```python
from build123d import *

# Parameters (mm, degrees)
SKETCH1_R           = 37
BOSS_EXTRUDE1_DEPTH = 3
SKETCH1_3_R         = 30
SKETCH1_3_R_2       = 14
BOSS_EXTRUDE2_DEPTH = 29
CUT_EXTRUDE1_START  = -4
SKETCH2_R           = 25
SKETCH2_R_2         = 23.5
CUT_EXTRUDE1_DEPTH  = 4
SKETCH3_R           = 4
SKETCH3_R_2         = 2
CUT_EXTRUDE2_DEPTH  = 4


with BuildPart() as part:
    # Sketch1 → Boss-Extrude1 (new body)
    with BuildSketch(Plane(origin=(0, 0, 0), x_dir=(1, 0, 0), z_dir=(0, 1, 0))):
        with Locations(Location((0, 0, 0), (0, 0, 270))):
            Circle(SKETCH1_R)
    extrude(amount=BOSS_EXTRUDE1_DEPTH)

    # Sketch1<3> → Boss-Extrude2 (add)
    with BuildSketch(Plane(origin=(0, 0, 0), x_dir=(1, 0, 0), z_dir=(0, 1, 0))):
        with Locations(Location((0, 0, 0), (0, 0, 90))):
            Circle(SKETCH1_3_R)
        with Locations(Location((0, 0, 0), (0, 0, 90))):
            Circle(SKETCH1_3_R_2, mode=Mode.SUBTRACT)
    extrude(amount=BOSS_EXTRUDE2_DEPTH)

    # Sketch2 → Cut-Extrude1 (cut)
    # profile 1 of 10: a face of its own
    with BuildSketch(Plane(origin=(0, 29, 0), x_dir=(1, 0, 0), z_dir=(0, 1, 0)).offset(CUT_EXTRUDE1_START)):
        with Locations(Location((0, 0, 0), (0, 0, 270))):
            Circle(SKETCH2_R)
        Circle(SKETCH2_R_2, mode=Mode.SUBTRACT)
    # profile 2 of 10: a face of its own
    with BuildSketch(Plane(origin=(0, 29, 0), x_dir=(1, 0, 0), z_dir=(0, 1, 0)).offset(CUT_EXTRUDE1_START)):
        with BuildLine():
            ThreePointArc((24.954959427, 1.5), (0, 25), (-24.954959427, 1.5))
            Line((-24.954959427, 1.5), (-23.452078799, 1.5))
            ThreePointArc((-23.452078799, 1.5), (0, 23.5), (23.452078799, 1.5))
            Line((23.452078799, 1.5), (24.954959427, 1.5))
        make_face()
    # profile 3 of 10: a face of its own
    with BuildSketch(Plane(origin=(0, 29, 0), x_dir=(1, 0, 0), z_dir=(0, 1, 0)).offset(CUT_EXTRUDE1_START)):
        with BuildLine():
            ThreePointArc((-24.954959427, 1.5), (-25, 0), (-24.954959427, -1.5))
            Line((-24.954959427, -1.5), (-23.452078799, -1.5))
            ThreePointArc((-23.452078799, -1.5), (-23.5, 0), (-23.452078799, 1.5))
            Line((-23.452078799, 1.5), (-24.954959427, 1.5))
        make_face()
    # profile 4 of 10: a face of its own
    with BuildSketch(Plane(origin=(0, 29, 0), x_dir=(1, 0, 0), z_dir=(0, 1, 0)).offset(CUT_EXTRUDE1_START)):
        with BuildLine():
            Line((23.452078799, -1.5), (24.954959427, -1.5))
            ThreePointArc((24.954959427, -1.5), (24.98873732, -0.750338033), (25, 0))
            ThreePointArc((25, 0), (24.98873732, 0.750338033), (24.954959427, 1.5))
            Line((24.954959427, 1.5), (23.452078799, 1.5))
            ThreePointArc((23.452078799, 1.5), (23.488016644, 0.750382643), (23.5, 0))
            ThreePointArc((23.5, 0), (23.488016644, -0.750382643), (23.452078799, -1.5))
        make_face()
    # profile 5 of 10: a face of its own
    with BuildSketch(Plane(origin=(0, 29, 0), x_dir=(1, 0, 0), z_dir=(0, 1, 0)).offset(CUT_EXTRUDE1_START)):
        with BuildLine():
            ThreePointArc((-23.452078799, 1.5), (-23.5, 0), (-23.452078799, -1.5))
            Line((-23.452078799, -1.5), (-13.919410907, -1.5))
            ThreePointArc((-13.919410907, -1.5), (-14, 0), (-13.919410907, 1.5))
            Line((-13.919410907, 1.5), (-23.452078799, 1.5))
        make_face()
    # profile 6 of 10: a face of its own
    with BuildSketch(Plane(origin=(0, 29, 0), x_dir=(1, 0, 0), z_dir=(0, 1, 0)).offset(CUT_EXTRUDE1_START)):
        with BuildLine():
            Line((13.919410907, -1.5), (23.452078799, -1.5))
            ThreePointArc((23.452078799, -1.5), (23.488016644, -0.750382643), (23.5, 0))
            ThreePointArc((23.5, 0), (23.488016644, 0.750382643), (23.452078799, 1.5))
            Line((23.452078799, 1.5), (13.919410907, 1.5))
            ThreePointArc((13.919410907, 1.5), (13.979838209, 0.751081654), (14, 0))
            ThreePointArc((14, 0), (13.979838209, -0.751081654), (13.919410907, -1.5))
        make_face()
    # profile 7 of 10: a face of its own
    with BuildSketch(Plane(origin=(0, 29, 0), x_dir=(1, 0, 0), z_dir=(0, 1, 0)).offset(CUT_EXTRUDE1_START)):
        with BuildLine():
            ThreePointArc((-23.452078799, 1.5), (-23.5, 0), (-23.452078799, -1.5))
            Line((-23.452078799, -1.5), (-13.919410907, -1.5))
            ThreePointArc((-13.919410907, -1.5), (-14, 0), (-13.919410907, 1.5))
            Line((-13.919410907, 1.5), (-23.452078799, 1.5))
        make_face()
    # profile 8 of 10: a face of its own
    with BuildSketch(Plane(origin=(0, 29, 0), x_dir=(1, 0, 0), z_dir=(0, 1, 0)).offset(CUT_EXTRUDE1_START)):
        with BuildLine():
            Line((13.919410907, -1.5), (23.452078799, -1.5))
            ThreePointArc((23.452078799, -1.5), (23.488016644, -0.750382643), (23.5, 0))
            ThreePointArc((23.5, 0), (23.488016644, 0.750382643), (23.452078799, 1.5))
            Line((23.452078799, 1.5), (13.919410907, 1.5))
            ThreePointArc((13.919410907, 1.5), (13.979838209, 0.751081654), (14, 0))
            ThreePointArc((14, 0), (13.979838209, -0.751081654), (13.919410907, -1.5))
        make_face()
    # profile 9 of 10: a face of its own
    with BuildSketch(Plane(origin=(0, 29, 0), x_dir=(1, 0, 0), z_dir=(0, 1, 0)).offset(CUT_EXTRUDE1_START)):
        with BuildLine():
            ThreePointArc((-24.954959427, 1.5), (-25, 0), (-24.954959427, -1.5))
            Line((-24.954959427, -1.5), (-23.452078799, -1.5))
            ThreePointArc((-23.452078799, -1.5), (-23.5, 0), (-23.452078799, 1.5))
            Line((-23.452078799, 1.5), (-24.954959427, 1.5))
        make_face()
    # profile 10 of 10: a face of its own
    with BuildSketch(Plane(origin=(0, 29, 0), x_dir=(1, 0, 0), z_dir=(0, 1, 0)).offset(CUT_EXTRUDE1_START)):
        with BuildLine():
            Line((23.452078799, -1.5), (24.954959427, -1.5))
            ThreePointArc((24.954959427, -1.5), (24.98873732, -0.750338033), (25, 0))
            ThreePointArc((25, 0), (24.98873732, 0.750338033), (24.954959427, 1.5))
            Line((24.954959427, 1.5), (23.452078799, 1.5))
            ThreePointArc((23.452078799, 1.5), (23.488016644, 0.750382643), (23.5, 0))
            ThreePointArc((23.5, 0), (23.488016644, -0.750382643), (23.452078799, -1.5))
        make_face()
    extrude(amount=CUT_EXTRUDE1_DEPTH, mode=Mode.SUBTRACT)

    # Sketch3 → Cut-Extrude2 (cut)
    with BuildSketch(Plane.XZ):
        with Locations(Location((0, 0, 0), (0, 0, 270))):
            Circle(SKETCH3_R)
        with Locations(Location((-8, 0, 0), (0, 0, 270))):
            Circle(SKETCH3_R_2)
        with Locations(Location((0, 8, 0), (0, 0, 270))):
            Circle(SKETCH3_R_2)
        with Locations(Location((8, 0, 0), (0, 0, 270))):
            Circle(SKETCH3_R_2)
        with Locations(Location((0, -8, 0), (0, 0, 270))):
            Circle(SKETCH3_R_2)
    extrude(amount=-CUT_EXTRUDE2_DEPTH, mode=Mode.SUBTRACT)


solid = part.part
```
The model under review builds one solid part; all positions refer to its coordinate system, in mm. A direction names the side the tool comes from. Give positions to 0.01 mm unless a question says otherwise; leave off trailing zeros. Write each loop counter-clockwise with the first axis right and the second up, starting at its lowest first coordinate (ties: lowest second). Pieces come first, ordered by that corner, then holes. Notation, with made-up numbers: (54, 2.5) -> (86, 2.5) arc R12 ccw to (86, 20.5) -> close; hole circle Ø10 at (32, 61.25). An arc over 180 degrees is marked (long way). Put each result on its own line as item: value.
(1) We need section C-C, the plane y = 19.5. Give the boundary of the cut face in (x, z), and give its area (3 significant figures).
Results are:
outline: circle Ø60 at (0, 0); hole circle Ø28 at (0, 0)
area: 2,210 mm²
(2) We need section D-D, the plane x = -8. Give the boundary of the cut face in (y, z), and give its area (3 significant figures).
Results are:
outline: (0, -36.12) -> (3, -36.12) -> (3, -28.91) -> (29, -28.91) -> (29, -23.69) -> (25, -23.69) -> (25, -22.1) -> (29, -22.1) -> (29, -11.49) -> (3, -11.49) -> (3, -2) -> (0, -2) -> close; (0, 2) -> (3, 2) -> (3, 11.49) -> (29, 11.49) -> (29, 22.1) -> (25, 22.1) -> (25, 23.69) -> (29, 23.69) -> (29, 28.91) -> (3, 28.91) -> (3, 36.12) -> (0, 36.12) -> close
area: 1,100 mm²
(3) The part is to be moulded in two halves that separate along X. For faces 3 (the cylindrical face through (-0.496, 26.972, 23.495)), 4 (the flat face through (-25, 29, 7)), 5 (the cylindrical face through (-14.17, 1.48, 34.18)), say which applies: pulls with the +X half, pulls with the -X half, needs draft (parallel to the pull), parting line crosses it, or undercut.
Results are:
face 3: undercut
face 4: needs draft
face 5: parting line crosses it
(4) For pin 1 Ø5 at (y, z) = (13.5, -16.5) entering from -X; pin 2 Ø8.5 at (x, z) = (-0.5, 3.5) entering from +Y; pin 3 Ø1 at (x, y) = (19, 20) entering from +Z, all flat-tipped, find the tip position at first contact; note any pin that passes through.
Results are:
pin 1: x = -26.53
pin 2: y = 3
pin 3: z = 23.62
(5) To check wall thickness, follow probe 1 along X at (y, z) = (0.7, 0); probe 2 along X at (y, z) = (15.5, 0); probe 3 along Z at (x, y) = (-4, 25.75). State the ranges of each line that lie inside material, in increasing order. Write a range as from..to.
Results are:
probe 1: -37..-10, -6..-4, 4..6, 10..37
probe 2: -30..-14, 14..30
probe 3: -29.73..-24.68, -23.16..-13.42, 13.42..23.16, 24.68..29.73
(6) We need section B-B, the plane x = 0. State how many separate pieces and enclosed holes the cut face has, and give its area (3 significant figures).
Results are:
separate pieces: 4
enclosed holes: 0
area: 994 mm²
(7) Tool access review of faces 1 (the cylindrical face through (0, 1, -6)), 2 (the flat face through (30.3, 3, -0.2)): name each direction out of +Z, -Z, +X, -X, +Y, -Y from which nothing blocks a thin tool from reaching the whole face with its end or side.
Results are:
face 1: +Y, -Y
face 2: +Y
(8) We need section A-A, the plane z = -8. Give the boundary of the cut face in (x, y).
Results are:
outline: (-36.12, 0) -> (-2, 0) -> (-2, 3) -> (-11.49, 3) -> (-11.49, 29) -> (-22.1, 29) -> (-22.1, 25) -> (-23.69, 25) -> (-23.69, 29) -> (-28.91, 29) -> (-28.91, 3) -> (-36.12, 3) -> close; (2, 0) -> (36.12, 0) -> (36.12, 3) -> (28.91, 3) -> (28.91, 29) -> (23.69, 29) -> (23.69, 25) -> (22.1, 25) -> (22.1, 29) -> (11.49, 29) -> (11.49, 3) -> (2, 3) -> close
